Can you work these out from the model? Positions are in its coordinate system, mm. Face numbers are marked on the shaded views. A direction names the side the tool comes from. Give positions to 0.01 mm unless a question says otherwise; leave off trailing zeros. Loops run counter-clockwise (first coordinate to the right, second up) from the corner with the lowest first, then second, coordinate; pieces in that order, holes last. Notation, with made-up numbers: M 15.25,24.5 L 63.25,24.5 A13 ccw 63.25,48.5 Z; hole C -32.5,-31.5 d10. An arc over 180 degrees is marked long. Use CSV: the item, a comma, the result in double quotes.
Autodesk Inventor part; units mm, degrees
ref_plane "YZ Plane" through (0, 0, 0) normal (1, 0, 0) x (0, 1, 0)
ref_plane "XZ Plane" through (0, 0, 0) normal (0, 1, 0) x (-1, 0, 0)
ref_plane "XY Plane" through (0, 0, 0) normal (0, 0, 1) x (1, 0, 0)
sketch "Sketch1" plane through (0, 0, 0) normal (0, 1, 0) x (-1, 0, 0)
  line L0 (0, 0) -> (-25.4, 0)
  line L1 (-25.4, 0) -> (-25.4, -25.4)
  line L2 (-25.4, -25.4) -> (0, -25.4)
  line L3 (0, -25.4) -> (0, 0)
  line L4 (-3.175, -3.175) -> (-22.225, -3.175)
  line L5 (-22.225, -3.175) -> (-22.225, -22.225)
  line L6 (-22.225, -22.225) -> (-3.175, -22.225)
  line L7 (-3.175, -22.225) -> (-3.175, -3.175)
  dimension "d0" = 25.4
  dimension "d1" = 25.4
  dimension "d2" = 19.05
  dimension "d3" = 19.05
  dimension "d4" = 3.175
  dimension "d5" = 3.175
extrude "Extrusion1" add sketch "Sketch1" along normal blind 155.575
sketch "Sketch2" plane through (0, 0, 0) normal (0, 0, 1) x (1, 0, 0)
  line L0 (0, 0) -> (25.4, 0)
  line L1 (0, 155.575) -> (25.4, 155.575)
  line L2 (0, 0) -> (0, 155.575)
  point P0 (12.7, 142.875)
  point P1 (12.7, 12.7)
  dimension "d8" = 12.7
  dimension "d9" = 12.7
  dimension "d10" = 12.7
  dimension "d11" = 12.7
hole "Hole1" at (12.7, 142.875, 0) at (12.7, 12.7, 0) direction (0, 0, -1) diameter 6.35 end through all
sketch "Sketch3" plane through (25.4, 0, 0) normal (1, 0, 0) x (0, 0, -1)
  line L0 (0, 0) -> (25.4, 0)
  line L1 (0, 0) -> (0, 155.575)
  point P0 (12.7, 38.1)
  dimension "d21" = 12.7
  dimension "d22" = 38.1
hole "Hole2" at (25.4, 38.1, -12.7) direction (-1, 0, 0) diameter 9.525 end through all
sketch "Sketch6" plane through (25.4, 0, 0) normal (1, 0, 0) x (0, 0, -1)
  circle A0 centre (12.7, 38.1) radius 4.7625
  circle A1 centre (12.7, 38.1) radius 6.35
  dimension "d54" = 12.7
extrude "Extrusion2" cut sketch "Sketch6" against normal blind 12.7
properties part number "1x1 vertical" material "Aluminum 6061"
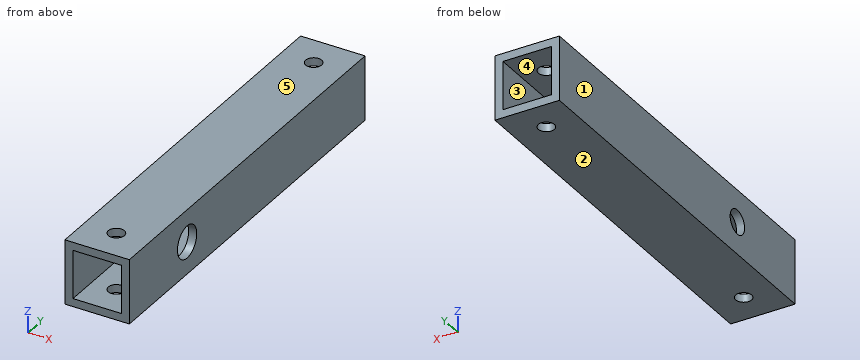
Q1. Please list where these lines run through material, in increasing order: L1, parallel to Y at x = 12.7, z = -24.2 (3 decimals); L2, parallel to X at y = 144, z = -11 (3 decimals); L3, parallel to Y at x = 1, z = -12.7 (1 decimal). Write a range as from..to.
Model answer:
L1,"0..9.525, 15.875..139.7, 146.05..155.575"
L2,"0..3.175, 22.225..25.4"
L3,"0..33.3, 42.9..155.6"
Q2. I want a section at C-C, the plane y = 12.7. Please give me the cut outline in (x, z) (3 decimals).
Model answer:
outline,"M 0,-25.4 L 9.525,-25.4 L 9.525,-22.225 L 3.175,-22.225 L 3.175,-3.175 L 9.525,-3.175 L 9.525,0 L 0,0 Z; M 15.875,-25.4 L 25.4,-25.4 L 25.4,0 L 15.875,0 L 15.875,-3.175 L 22.225,-3.175 L 22.225,-22.225 L 15.875,-22.225 Z"
Q3. I want a section at A-A, the plane x = 12.7. Please give me the cut outline in (y, z) (3 decimals), then the cut area to 3 significant figures.
Model answer:
outline,"M 0,-25.4 L 9.525,-25.4 L 9.525,-22.225 L 0,-22.225 Z; M 0,-3.175 L 9.525,-3.175 L 9.525,0 L 0,0 Z; M 15.875,-25.4 L 139.7,-25.4 L 139.7,-22.225 L 15.875,-22.225 Z; M 15.875,-3.175 L 139.7,-3.175 L 139.7,0 L 15.875,0 Z; M 146.05,-25.4 L 155.575,-25.4 L 155.575,-22.225 L 146.05,-22.225 Z; M 146.05,-3.175 L 155.575,-3.175 L 155.575,0 L 146.05,0 Z"
area,"907 mm2"
Q4. I want a section at D-D, the plane x = 19.5. Please give me the cut outline in (y, z) (3 decimals).
Model answer:
outline,"M 0,-25.4 L 155.575,-25.4 L 155.575,-22.225 L 0,-22.225 Z; M 0,-3.175 L 155.575,-3.175 L 155.575,0 L 0,0 Z"
Q5. For the marked faces 4 and 5, which set-ups out of +Z, -Z, +X, -X, +Y, -Y let a thin tool reach every point of the face, with its end or its side?
Model answer:
face 4,"+Y, -Y"
face 5,"+Z, +X, -X, +Y, -Y"
Q6. I want a section at B-B, the plane z = -12.7. State how many separate pieces and enclosed holes the cut face has, then the cut area to 3 significant figures.
Model answer:
separate pieces,"4"
enclosed holes,"0"
area,"917 mm2"
Q7. If we mould it in two halves opening along X, with no side actions, what happens to the marked faces 1, 2 and 3? For each: released by +X, released by -X, zero draft, split by the parting line, or undercut.
Model answer:
face 1,"released by -X"
face 2,"zero draft"
face 3,"undercut"
